Here's how the part is built. I have some questions about the finished solid (model axes, mm). A direction names the side the tool comes from. Give positions to 0.01 mm unless a question says otherwise; leave off trailing zeros. Loops run counter-clockwise (first coordinate to the right, second up) from the corner with the lowest first, then second, coordinate; pieces in that order, holes last. Notation, with made-up numbers: (41.5, 69) -> (58.5, 69) arc R19 ccw to (58.5, 90) -> close; hole circle Ø9 at (14.5, -15). An arc over 180 degrees is marked (long way). Answer in a Markdown table with one row per item. Add a question column.
Item 1: If we section it at B-B (y = 0): Write out the boundary of the cut face in (x, z), then the cut area to 3 significant figures.
Item 2: Which directions (+Z, -Z, +X, -X, +Y, -Y) give clear straight access to the entire face, cutting with the end or side of a thin tool? Please do faces 1 (the face through (-1.5, 4, 2)), 2 (the face through (4, -2, 0)), 3 (the face through (3.5, 21, 2)), 4 (the face through (-3.5, 21, 2)).
Item 3: If I drill on line 1 (Y direction, x = 0, z = 0.7); line 2 (X direction, y = -1.8, z = 0.95); line 3 (Y direction, x = 1, z = 1.35), over which ranges is the centre line in solid material (lowest first)?
Item 4: If we section it at D-D (y = 11): Write out the boundary of the cut face in (x, z).
Item 5: For P1, Ø0.9, axis at y = 8.5, z = 2.5, coming from the +X side; P2, Ø1.4, axis at y = 20.5, z = 2, coming from the +X side; P3, Ø1.6, axis at y = 6, z = 1.5, coming from the +X side, each with a flat end and sliding along its axis, tell me the tip position at first contact or that it passes through.
Item 6: We'd pull the mould along X, two halves only. Please class faces 5 (the face through (-3, 8, 2)), 6 (the face through (0, 25, 2)), 7 (the face through (4, -2, 3.3)): released by +X, released by -X, zero draft, split by the parting line, or undercut.
Item 7: If we section it at A-A (x = 0): Write out the boundary of the cut face in (y, z), then the cut area to 3 significant figures.
Item 8: If we section it at C-C (z = 0.75): Write out the boundary of the cut face in (x, y).
```python
from build123d import *

# Parameters (mm, degrees)
EXTRUDE_DEPTH   = 3.3
SKETCH001_R     = 1.5
POCKET_DEPTH    = 3.301
POCKET001_DEPTH = 3.301


with BuildPart() as part:
    # Sketch → Extrude (new body)
    with BuildSketch(Plane.XY):
        with BuildLine():
            ThreePointArc((3.5, 21.5), (0, 25), (-3.5, 21.5))
            Line((-3.5, 21.5), (-3.5, 19.691369))
            ThreePointArc((-3.5, 19.691369), (0, -20), (3.5, 19.691369))
            Line((3.5, 19.691369), (3.5, 21.5))
        make_face()
    extrude(amount=EXTRUDE_DEPTH)

    # Sketch001 (on Face6 of Extrude) → Pocket (cut, through all)
    with BuildSketch(Plane.XY.offset(3.3)):
        with Locations((0, 21.5)):
            Circle(SKETCH001_R)
    extrude(amount=-POCKET_DEPTH, mode=Mode.SUBTRACT)

    # Sketch002 (on Face6 of BaseFeature) → Pocket001 (cut, through all)
    with BuildSketch(Plane.XY.offset(3.3)):
        with BuildLine():
            Line((-1.5, 13), (-1.5, -5))
            ThreePointArc((-1.5, -5), (0, -6.5), (1.5, -5))
            Line((1.5, 13), (1.5, -5))
            ThreePointArc((1.5, 13), (0, 14.5), (-1.5, 13))
        make_face()
        with BuildLine():
            ThreePointArc((-3, 6.81895), (0, -10.926133), (3, 6.81895))
            Line((3, 9.81895), (3, 6.81895))
            ThreePointArc((-3, 9.81895), (0, -13.8), (3, 9.81895))
            Line((-3, 6.81895), (-3, 9.81895))
        make_face()
    extrude(amount=-POCKET001_DEPTH, mode=Mode.SUBTRACT)


solid = part.part
```
Recorded:
| question | item | result |
|---|---|---|
| 1 | outline | (-20, 0) -> (-11.86, 0) -> (-11.86, 3.3) -> (-20, 3.3) -> close; (-8.95, 0) -> (-1.5, 0) -> (-1.5, 3.3) -> (-8.95, 3.3) -> close; (1.5, 0) -> (8.95, 0) -> (8.95, 3.3) -> (1.5, 3.3) -> close; (11.86, 0) -> (20, 0) -> (20, 3.3) -> (11.86, 3.3) -> close |
| 1 | area | 103 mm^2 |
| 2 | face 1 | +Z, -Z |
| 2 | face 2 | -Z, +X, -X, +Y, -Y |
| 2 | face 3 | +Z, -Z, +X, +Y |
| 2 | face 4 | +Z, -Z, -X, +Y |
| 3 | line 1 | y = -20 to -13.8, -10.93 to -6.5, 14.5 to 20, 23 to 25 |
| 3 | line 2 | x = -19.92 to -12, -9.13 to -1.5, 1.5 to 9.13, 12 to 19.92 |
| 3 | line 3 | y = -19.97 to -13.76, -10.87 to -6.12, 14.12 to 20.38, 22.62 to 24.85 |
| 4 | outline | (-16.7, 0) -> (-1.5, 0) -> (-1.5, 3.3) -> (-16.7, 3.3) -> close; (1.5, 0) -> (16.7, 0) -> (16.7, 3.3) -> (1.5, 3.3) -> close |
| 5 | P1 | stops at x = 18.31 |
| 5 | P2 | stops at x = 3.5 |
| 5 | P3 | stops at x = 19.31 |
| 6 | face 5 | undercut |
| 6 | face 6 | split by the parting line |
| 6 | face 7 | zero draft |
| 7 | outline | (-20, 0) -> (-13.8, 0) -> (-13.8, 3.3) -> (-20, 3.3) -> close; (-10.93, 0) -> (-6.5, 0) -> (-6.5, 3.3) -> (-10.93, 3.3) -> close; (14.5, 0) -> (20, 0) -> (20, 3.3) -> (14.5, 3.3) -> close; (23, 0) -> (25, 0) -> (25, 3.3) -> (23, 3.3) -> close |
| 7 | area | 59.8 mm^2 |
| 8 | outline | (-3.5, 19.69) arc R20 ccw (long way) to (3.5, 19.69) -> (3.5, 21.5) arc R3.5 ccw to (-3.5, 21.5) -> close; hole (-3, 6.82) -> (-3, 9.82) arc R12 ccw (long way) to (3, 9.82) -> (3, 6.82) arc R9.13 cw (long way) to start; hole (-1.5, -5) arc R1.5 ccw to (1.5, -5) -> (1.5, 13) arc R1.5 ccw to (-1.5, 13) -> close; hole circle Ø3 at (0, 21.5) |
